The listing builds one solid part. Answer for the finished solid, in the listing's coordinates (mm). Face numbers are marked on the shaded views. A direction names the side the tool comes from. Coordinates: 2 decimals unless noted, no trailing zeros. Loops run counter-clockwise (first coordinate to the right, second up) from the corner with the lowest first, then second, coordinate; pieces in that order, holes last. Notation, with made-up numbers: M 75,-20 L 87,-20 A17 ccw 87,9 Z; hole C -39.5,-28 d2. An arc over 180 degrees is marked long. Answer as a JSON object with one key per item and string values. Group by question number.
1. A cutting plane is placed at A-A on y = 0. Give the vertices of the cut face in (x, z) (3 decimals).
2. Given pin 1 (2 mm diameter, centred on x = 13.45, y = 10.38, fed in from -Z); pin 2 (2.5 mm diameter, centred on y = -2.5, z = 1, fed in from +X) (3 decimals), each flat-ended and moving along its own axis, determine where each tip first touches the part or whether it passes through.
3. Straight lines are drawn through the part: L1, parallel to X at y = -13, z = 2.8 (3 decimals); L2, parallel to Y at x = 12, z = 1.3; L3, parallel to Y at x = -15, z = 3.4. For each, find the intervals that lie inside material, in ascending order.
4. For the marked faces 1 and 2, determine the directions among +Z, -Z, +X, -X, +Y, -Y from which every point of the face is accessible in a straight line to the end or side of a thin tool.
5. A cutting plane is placed at B-B on z = 1.7. Give the vertices of the cut face in (x, y) (3 decimals).
from build123d import *

# Parameters (mm, degrees)
BOSS_EXTRUDE1_DEPTH = 2.4
SKETCH2_W           = 33.15
SKETCH2_H           = 36
SKETCH2_R           = 11.75
SKETCH2_R_2         = 0.822021887
SKETCH2_R_3         = 0.927108541
BOSS_EXTRUDE2_DEPTH = 2.33
CHAMFER1_SIZE       = 1.2
CHAMFER1_SIZE2      = 2.078460969
SKETCH3_R           = 0.8
CUT_EXTRUDE1_DEPTH  = 5.8
CHAMFER2_SIZE       = 1.2


with BuildPart() as part:
    # Sketch1 → Boss-Extrude1 (new body)
    with BuildSketch(Plane.XY):
        Polygon((-16.575, -18), (16.575, -18), (16.575, -13.05), (-14.975, -13.05), (-14.975, 13.05), (16.575, 13.05), (16.575, 18), (-16.575, 18), align=None)
    extrude(amount=BOSS_EXTRUDE1_DEPTH)

    # Sketch2 → Boss-Extrude2 (add)
    with BuildSketch(Plane.XY.offset(2.4)):
        Rectangle(SKETCH2_W, SKETCH2_H)
        with Locations((0.965, 0)):
            Circle(SKETCH2_R, mode=Mode.SUBTRACT)
        with Locations((13.452978113, 10.377978113)):
            Circle(SKETCH2_R_2, mode=Mode.SUBTRACT)
        with Locations((-11.747891459, -10.272891459)):
            Circle(SKETCH2_R_3, mode=Mode.SUBTRACT)
    extrude(amount=BOSS_EXTRUDE2_DEPTH)

    # Chamfer1
    chamfer1_edges = [part.edges().sort_by_distance(p)[0] for p in [
        (12.630956227, 10.377978113, 4.73),
        (-12.675, -10.272891459, 4.73),
    ]]
    chamfer1_side = [part.faces().sort_by_distance(p)[0] for p in [
        (0, 17.510620546, 4.73),
    ]]
    chamfer(chamfer1_edges, length=CHAMFER1_SIZE, length2=CHAMFER1_SIZE2, reference=chamfer1_side[0])

    # Sketch3 → Cut-Extrude1 (cut)
    with BuildSketch(Plane.XY.offset(4.73)):
        with Locations((-14.575, 16)):
            Circle(SKETCH3_R)
        with Locations(Location((14.575, 16, 0), (0, 0, 180))):
            Circle(SKETCH3_R)
        with Locations((-15.075, -13)):
            Circle(SKETCH3_R)
        with Locations(Location((15.075, -13, 0), (0, 0, 356.416678302))):
            Circle(SKETCH3_R)
    extrude(amount=-CUT_EXTRUDE1_DEPTH, mode=Mode.SUBTRACT)

    # Chamfer2
    # the kernel refuses this chamfer: 1.2 mm, written as the material it takes off along each edge
    with BuildSketch(Plane(origin=(14.575, 16, 4.73), x_dir=(-1, 0, 0), z_dir=(0, 1, 0))) as chamfer2_piece_1:
        Polygon((0.8 + CHAMFER2_SIZE, 0), (0.8, -CHAMFER2_SIZE), (0.8, 0), align=None)
    revolve(axis=Axis((14.575, 16, 4.73), (0, 0, 1)), mode=Mode.SUBTRACT)
    with BuildSketch(Plane(origin=(-15.075, -13, 4.73), x_dir=(1, 0, 0), z_dir=(0, -1, 0))) as chamfer2_piece_2:
        Polygon((0.8 + CHAMFER2_SIZE, 0), (0.8, -CHAMFER2_SIZE), (0.8, 0), align=None)
    revolve(axis=Axis((-15.075, -13, 4.73), (0, 0, 1)), mode=Mode.SUBTRACT)
    with BuildSketch(Plane(origin=(15.075, -13, 4.73), x_dir=(0.9980449639174719, -0.06249999999177853, 0), z_dir=(-0.06249999999177853, -0.9980449639174719, 0))) as chamfer2_piece_3:
        Polygon((0.8 + CHAMFER2_SIZE, 0), (0.8, -CHAMFER2_SIZE), (0.8, 0), align=None)
    revolve(axis=Axis((15.075, -13, 4.73), (0, 0, 1)), mode=Mode.SUBTRACT)
    with BuildSketch(Plane(origin=(-14.575, 16, 4.73), x_dir=(1, 0, 0), z_dir=(0, -1, 0))) as chamfer2_piece_4:
        Polygon((0.8 + CHAMFER2_SIZE, 0), (0.8, -CHAMFER2_SIZE), (0.8, 0), align=None)
    revolve(axis=Axis((-14.575, 16, 4.73), (0, 0, 1)), mode=Mode.SUBTRACT)


solid = part.part
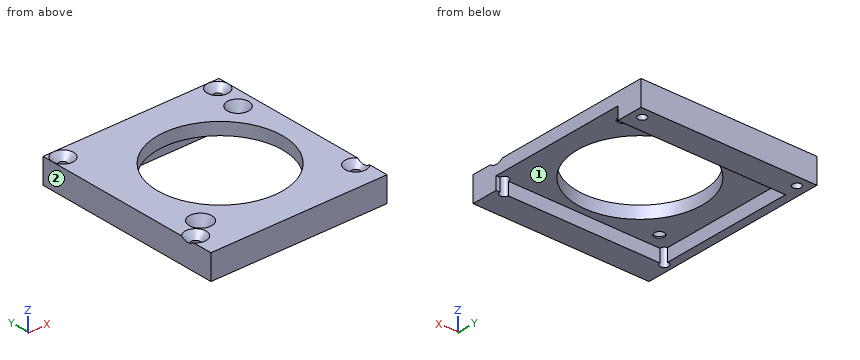
From the geometry:
{
 "1": {"outline": "M -16.575,0 L -14.975,0 L -14.975,2.4 L -10.785,2.4 L -10.785,4.73 L -16.575,4.73 Z; M 12.715,2.4 L 16.575,2.4 L 16.575,4.73 L 12.715,4.73 Z"},
 "2": {"pin 1": "stops at z = 2.4", "pin 2": "stops at x = -14.975"},
 "3": {"L1": "x = -16.575 to -15.875, -14.275 to 14.275, 15.875 to 16.575", "L2": "y = -18 to -13.05, 13.05 to 18", "L3": "y = -18 to -13.8, -12.2 to 15.32, 16.68 to 18"},
 "4": {"face 1": "-Z, +X", "face 2": "+Z, -Z, -X, +Y, -Y"},
 "5": {"outline": "M -16.575,-18 L 16.575,-18 L 16.575,-13.05 L 15.873,-13.05 A0.8 cw 14.277,-13.05 L -14.277,-13.05 A0.8 cw long -14.975,-12.206 L -14.975,13.05 L 16.575,13.05 L 16.575,18 L -16.575,18 Z; hole C -14.575,16 d1.6; hole C 14.575,16 d1.6"}
}
